Autodesk Inventor part; units mm, degrees
ref_plane "YZ Plane" through (0, 0, 0) normal (1, 0, 0) x (0, 1, 0)
ref_plane "XZ Plane" through (0, 0, 0) normal (0, 1, 0) x (-1, 0, 0)
ref_plane "XY Plane" through (0, 0, 0) normal (0, 0, 1) x (1, 0, 0)
ref_plane "작업 평면1" through (0, 0, 0) normal (0, 0, 1) x (1, 0, 0)
sketch "스케치1" plane through (0, 0, 0) normal (0, 0, 1) x (1, 0, 0)
  line L0 (-20.1, 0.025) -> (-14.5, 0.025)
  line L1 (-20.1, -44.6) -> (-20.1, 8.5)
  line L2 (20.1, 0.025) -> (14.5, 0.025)
  line L3 (20.1, 8.5) -> (20.1, -44.6)
  circle A0 centre (17.3, 4) radius 1.45
  circle A1 centre (-17.3, 4) radius 1.35
  circle A2 centre (-17.3, 4) radius 1.45
  circle A3 centre (17.3, 4) radius 1.55
  line L4 (14.9, 0.025) -> (14.9, 15.025)
  line L5 (-14.9, 15.025) -> (-14.9, 0.025)
  line L6 (-20.1, 0.025) -> (-20.1, 15.025)
  line L7 (20.1, 0.025) -> (20.1, 15.025)
  line L8 (-20.1, 15.025) -> (20.1, 15.025)
  line L9 (-20.1, 0.025) -> (-14.9, 0.025)
  line L10 (14.9, 0.025) -> (20.1, 0.025)
  line L11 (-14.9, 0.025) -> (-14.9, 10.025)
  line L12 (-14.9, 10.025) -> (14.9, 10.025)
  line L13 (14.9, 0.025) -> (20.1, 0.025)
  point P0 (0, 0)
  point P1 (-20.1, 8.5)
  point P2 (-14.9, 0.025)
  dimension "d0" = 0.1
  dimension "d1" = 0.1
  dimension "d4" = 15
  dimension "d5" = 15
  dimension "d9" = 10
extrude "돌출1" add sketch "스케치1" along normal blind 6 contours L1 L6 L8 L5 L0 | L5 L8 L4 L12 | L4 L8 L7 L3 L2
sketch "스케치5" plane through (0, 0, 6) normal (0, 0, 1) x (1, 0, 0)
  line L0 (15, -50.5) -> (11.5, -50.5)
  line L1 (15, -50.5) -> (20.1, -44.5)
  line L2 (20.1, -44.5) -> (20.1, 8.6)
  line L3 (20.1, 8.6) -> (15, 14.6)
  line L4 (15, 14.6) -> (-15, 14.6)
  line L5 (-15, 14.6) -> (-20.1, 8.6)
  line L6 (-20.1, 8.6) -> (-20.1, -44.5)
  line L7 (-20.1, -44.5) -> (-15, -50.5)
  line L8 (-11.5, -50.5) -> (-15, -50.5)
  arc A0 (-14.5, -47.5) -> (-11.5, -50.5) centre (-11.5, -47.5) ccw
  line L9 (-14.5, 6) -> (-14.5, -47.5)
  arc A1 (-11.5, 9) -> (-14.5, 6) centre (-11.5, 6) ccw
  line L10 (11.5, 9) -> (-11.5, 9)
  arc A2 (14.5, 6) -> (11.5, 9) centre (11.5, 6) ccw
  line L11 (14.5, -47.5) -> (14.5, 6)
  arc A3 (11.5, -50.5) -> (14.5, -47.5) centre (11.5, -47.5) ccw
  circle A4 centre (-17.3, -40) radius 1.35
  circle A5 centre (-17.3, -18) radius 1.35
  circle A6 centre (-17.3, 4) radius 1.35
  circle A7 centre (-11, 11.8) radius 1.35
  circle A8 centre (17.3, -40) radius 1.35
  circle A9 centre (17.3, -18) radius 1.35
  circle A10 centre (17.3, 4) radius 1.35
  circle A11 centre (11, 11.8) radius 1.35
  line L12 (20.1, 15.025) -> (-20.1, 15.025)
  line L13 (-20.1, 15.025) -> (-20.1, 0.025)
  line L14 (-20.1, 0.025) -> (-14.9, 0.025)
  line L15 (-14.9, 0.025) -> (-14.9, 10.025)
  line L16 (-14.9, 10.025) -> (14.9, 10.025)
  line L17 (14.9, 10.025) -> (14.9, 0.025)
  line L18 (14.9, 0.025) -> (20.1, 0.025)
  line L19 (20.1, 0.025) -> (20.1, 15.025)
  circle A12 centre (17.3, 4) radius 1.55
  circle A13 centre (-17.3, 4) radius 1.45
  line L20 (-14.9, 15.025) -> (-26.9, 15.025)
  line L21 (-26.9, 15.025) -> (-26.9, -22.7435)
  line L22 (-26.9, -22.7435) -> (-14.9, -22.7435)
  line L23 (-14.9, -22.7435) -> (-14.9, 15.025)
  line L24 (14.9, 15.025) -> (26.9, 15.025)
  line L25 (26.9, 15.025) -> (26.9, -22.7435)
  line L26 (26.9, -22.7435) -> (14.9, -22.7435)
  line L27 (14.9, -22.7435) -> (14.9, 15.025)
  point P0 (0, 0)
  point P1 (0, -36)
  point P2 (20.1, 8.6)
  point P3 (20.1, -22.7435)
  point P4 (-20.1, -22.7435)
  point P5 (-20.1, 15.025)
  point P6 (20.1, 0.025)
  point P7 (-14.9, 0.025)
  dimension "d21" = 12
  dimension "d22" = 12
extrude "돌출5" add sketch "스케치5" against normal blind 6 contours L26 L27 L18 L2 | L23 L22 L6 L14
sketch "스케치12" plane through (0, 0, 6) normal (0, 0, 1) x (1, 0, 0)
  circle A0 centre (-17.3, -18) radius 1.35
  circle A1 centre (17.3, -18) radius 1.35
  line L0 (20.1, 15.025) -> (-20.1, 15.025)
  line L1 (-20.1, 15.025) -> (-20.1, -22.7435)
  line L2 (-20.1, -22.7435) -> (-14.9, -22.7435)
  line L3 (-14.9, -22.7435) -> (-14.9, 10.025)
  line L4 (-14.9, 10.025) -> (14.9, 10.025)
  line L5 (14.9, 10.025) -> (14.9, -22.7435)
  line L6 (14.9, -22.7435) -> (20.1, -22.7435)
  line L7 (20.1, -22.7435) -> (20.1, 15.025)
  circle A2 centre (17.3, 4) radius 1.55
  circle A3 centre (-17.3, 4) radius 1.45
  line L8 (0, 15.025) -> (-5, 15.025)
  line L9 (-5, 15.025) -> (-5, 21.025)
  line L10 (-5, 21.025) -> (0, 21.025)
  line L11 (0, 21.025) -> (0, 15.025)
  line L12 (0, 21.025) -> (5, 21.025)
  line L13 (5, 21.025) -> (5, 15.025)
  line L14 (5, 15.025) -> (0, 15.025)
  line L15 (0, 15.025) -> (0, 21.025)
  point P0 (0, 0)
  point P1 (5, 15.025)
  dimension "d53" = 5
  dimension "d54" = 6
  dimension "d55" = 5
  dimension "d56" = 6
extrude "돌출11" add sketch "스케치12" against normal blind 6 contours L0 L11 L12 L13 | L0 L9 L10 L11
sketch "스케치14" plane through (-20.1, 15.025, 6) normal (0, 1, 0) x (1, 0, 0)
  line L0 (5.2, 6) -> (5.2, 0)
  line L1 (15.1, 0) -> (15.1, 6)
  line L2 (15.1, 6) -> (0, 6)
  line L3 (0, 6) -> (0, 0)
  line L4 (15.1, 0) -> (0, 0)
  line L5 (25.1, 6) -> (25.1, 0)
  line L6 (40.2, 0) -> (25.1, 0)
  line L7 (40.2, 6) -> (40.2, 0)
  line L8 (40.2, 6) -> (25.1, 6)
  line L9 (35, 6) -> (35, 0)
  line L10 (0, 6) -> (2.6, 6)
  circle A0 centre (2.6, 3) radius 1.35
  line L11 (40.2, 6) -> (40.2, 0)
  line L12 (40.2, 6) -> (37.6, 6)
  circle A1 centre (37.6, 3) radius 1.35
  point P0 (20.1, 6)
  dimension "d59" = 6
  dimension "d60" = 5.2
  dimension "d61" = 2.6
  dimension "d62" = 2.7
  dimension "d63" = 2.6
  dimension "d64" = 2.7
extrude "돌출12" cut sketch "스케치14" against normal blind 6 contours A0 | A1
sketch "스케치16" plane through (-20.1, 15.025, 0) normal (-1, 0, 0) x (0, 0, 1)
  line L0 (0, 0) -> (0, -37.7685)
  line L1 (6, -37.7685) -> (0, -37.7685)
  line L2 (6, 0) -> (6, -37.7685)
  line L3 (0, 0) -> (6, 0)
  point P0 (0, -15.025)
extrude "돌출13" add sketch "스케치16" along normal blind 5
sketch "스케치18" plane through (20.1, 15.025, 6) normal (1, 0, 0) x (0, 0, -1)
  line L0 (6, 0) -> (6, -37.7685)
  line L1 (6, 0) -> (0, 0)
  line L2 (0, -37.7685) -> (0, 0)
  line L3 (0, -37.7685) -> (6, -37.7685)
  point P0 (6, -15.025)
extrude "돌출14" add sketch "스케치18" along normal blind 5
move faces "이동1" translate (0, 10, 0) faces at (8.7167, 15.025, 3) (1.6667, 21.025, 4) (-8.7167, 15.025, 3)
sketch "스케치19" plane through (0, 0, 6) normal (0, 0, 1) x (1, 0, 0)
  line L0 (-18.85, 9.025) -> (-16.15, 9.025)
  circle A0 centre (-17.3, 4) radius 1.45
  line L1 (-14.9, 10.025) -> (14.9, 10.025)
  line L2 (-14.9, 10.025) -> (14.9, 10.025)
  circle A1 centre (-17.3, -18) radius 1.35
  circle A2 centre (17.3, -18) radius 1.35
  line L3 (5, 25.025) -> (25.1, 25.025)
  line L4 (5, 25.025) -> (5, 31.025)
  line L5 (5, 31.025) -> (-5, 31.025)
  line L6 (-5, 31.025) -> (-5, 25.025)
  line L7 (-5, 25.025) -> (-25.1, 25.025)
  line L8 (-25.1, -22.7435) -> (-25.1, 25.025)
  line L9 (-25.1, -22.7435) -> (-14.9, -22.7435)
  line L10 (-14.9, -22.7435) -> (-14.9, 10.025)
  line L11 (-14.9, 10.025) -> (14.9, 10.025)
  line L12 (14.9, 10.025) -> (14.9, -22.7435)
  line L13 (14.9, -22.7435) -> (25.1, -22.7435)
  line L14 (25.1, 25.025) -> (25.1, -22.7435)
  circle A3 centre (17.3, 4) radius 1.55
  circle A4 centre (-17.3, 4) radius 1.45
  circle A5 centre (-17.3, -18) radius 1.35
  circle A6 centre (17.3, -18) radius 1.35
  line L15 (25.1, 25.025) -> (5, 25.025)
  line L16 (25.1, -22.7435) -> (25.1, 25.025)
  line L17 (14.9, -22.7435) -> (25.1, -22.7435)
  line L18 (14.9, 10.025) -> (14.9, -22.7435)
  line L19 (-14.9, 10.025) -> (14.9, 10.025)
  line L20 (-14.9, 10.025) -> (-14.9, -22.7435)
  line L21 (-14.9, -22.7435) -> (-25.1, -22.7435)
  line L22 (-25.1, 25.025) -> (-25.1, -22.7435)
  line L23 (-5, 25.025) -> (-25.1, 25.025)
  line L24 (-5, 25.025) -> (-5, 31.025)
  line L25 (-5, 31.025) -> (5, 31.025)
  line L26 (5, 31.025) -> (5, 25.025)
  circle A7 centre (17.3, 4) radius 1.55
  circle A8 centre (-17.3, 4) radius 1.45
  line L27 (-5, 25.025) -> (-5, 31.025)
  line L28 (-14.9, -22.7435) -> (-14.9, 10.025)
  line L29 (-14.9, 10.025) -> (-14.9, -22.7435)
  line L30 (-14.9, 10.025) -> (-14.9, -22.7435)
  line L31 (-14.9, -22.7435) -> (-14.9, 10.025)
  circle A9 centre (-17.3, -18) radius 1.35
  circle A10 centre (-17.3, -18) radius 1.35
  circle A11 centre (-17.3, -18) radius 1.35
  circle A12 centre (-17.3, -18) radius 1.35
  circle A13 centre (-17.3, 4) radius 1.45
  circle A14 centre (-17.3, 4) radius 1.45
  circle A15 centre (-17.3, 4) radius 1.45
  line L32 (-25.1, -22.7435) -> (-14.9, -22.7435)
  line L33 (-14.9, -22.7435) -> (-25.1, -22.7435)
  line L34 (-25.1, -22.7435) -> (-14.9, -22.7435)
  line L35 (-14.9, -22.7435) -> (-25.1, -22.7435)
  line L36 (-25.1, -22.7435) -> (-25.1, 25.025)
  line L37 (-25.1, 25.025) -> (-25.1, -22.7435)
  line L38 (-25.1, 25.025) -> (-25.1, -22.7435)
  line L39 (-25.1, -22.7435) -> (-25.1, 25.025)
  line L40 (14.9, -22.7435) -> (25.1, -22.7435)
  line L41 (14.9, 10.025) -> (14.9, -22.7435)
  line L42 (14.9, 10.025) -> (14.9, -22.7435)
  circle A16 centre (17.3, -18) radius 1.35
  circle A17 centre (17.3, -18) radius 1.35
  circle A18 centre (17.3, 4) radius 1.55
  circle A19 centre (17.3, 4) radius 1.55
  line L43 (16.15, 9.025) -> (18.85, 9.025)
  line L44 (14.9, -22.7435) -> (25.1, -22.7435)
  line L45 (25.1, 25.025) -> (25.1, -22.7435)
  line L46 (25.1, -22.7435) -> (25.1, 25.025)
  line L47 (25.1, -22.7435) -> (25.1, 25.025)
  line L48 (25.1, 25.025) -> (25.1, -22.7435)
  line L49 (-18.85, 9.025) -> (-16.15, 9.025)
  line L50 (-18.85, 25.025) -> (-16.15, 25.025)
  line L51 (-18.85, 9.025) -> (-16.15, 9.025)
  line L52 (-5, 25.025) -> (-25.1, 25.025)
  line L53 (-5, 25.025) -> (-25.1, 25.025)
  line L54 (-18.85, 25.025) -> (-16.15, 25.025)
  line L55 (-5, 25.025) -> (-25.1, 25.025)
  line L56 (-5, 25.025) -> (-25.1, 25.025)
  line L57 (-5, 31.025) -> (-5, 25.025)
  line L58 (5, 31.025) -> (-5, 31.025)
  line L59 (5, 31.025) -> (-5, 31.025)
  line L60 (-5, 31.025) -> (5, 31.025)
  line L61 (-5, 31.025) -> (-5, 25.025)
  line L62 (-5, 25.025) -> (-5, 31.025)
  line L63 (-18.85, 25.025) -> (-16.15, 25.025)
  line L64 (16.15, 25.025) -> (18.85, 25.025)
  line L65 (5, 25.025) -> (25.1, 25.025)
  line L66 (25.1, 25.025) -> (5, 25.025)
  line L67 (5, 31.025) -> (5, 25.025)
  line L68 (5, 25.025) -> (5, 31.025)
  line L69 (5, 25.025) -> (5, 31.025)
  line L70 (5, 31.025) -> (5, 25.025)
  line L71 (-5, 31.025) -> (5, 31.025)
  line L72 (14.9, -22.7435) -> (25.1, -22.7435)
  line L73 (14.9, -22.7435) -> (25.1, -22.7435)
  line L74 (-14.9, 10.025) -> (14.9, 10.025)
  line L75 (-14.9, 10.025) -> (14.9, 10.025)
  circle A20 centre (17.3, -18) radius 1.35
  circle A21 centre (17.3, -18) radius 1.35
  line L76 (14.9, 10.025) -> (14.9, -22.7435)
  line L77 (14.9, 10.025) -> (14.9, -22.7435)
  line L78 (16.15, 9.025) -> (18.85, 9.025)
  line L79 (16.15, 25.025) -> (18.85, 25.025)
  line L80 (16.15, 25.025) -> (18.85, 25.025)
  line L81 (5, 25.025) -> (25.1, 25.025)
  line L82 (25.1, 25.025) -> (5, 25.025)
  circle A22 centre (17.3, 4) radius 1.55
  circle A23 centre (17.3, 4) radius 1.55
  line L83 (16.15, 9.025) -> (18.85, 9.025)
  line L84 (-18.85, 25.025) -> (-18.85, 9.025)
  line L85 (-16.15, 25.025) -> (-16.15, 9.025)
  line L86 (16.15, 25.025) -> (16.15, 9.025)
  line L87 (18.85, 25.025) -> (18.85, 9.025)
  line L88 (-20.1, 15.925) -> (-14.9, 15.925)
  line L89 (-14.9, 15.925) -> (-14.9, 18.125)
  line L90 (-14.9, 18.125) -> (-20.1, 18.125)
  line L91 (-20.1, 18.125) -> (-20.1, 15.925)
  line L92 (-20.1, 15.925) -> (-14.9, 18.125) construction
  line L93 (-14.9, 15.925) -> (-20.1, 18.125) construction
  line L94 (14.9, 15.925) -> (20.1, 15.925)
  line L95 (20.1, 15.925) -> (20.1, 18.125)
  line L96 (20.1, 18.125) -> (14.9, 18.125)
  line L97 (14.9, 18.125) -> (14.9, 15.925)
  line L98 (14.9, 15.925) -> (20.1, 18.125) construction
  line L99 (20.1, 15.925) -> (14.9, 18.125) construction
  point P0 (0, 0)
  point P1 (-17.5, 17.025)
  point P2 (17.5, 17.025)
  dimension "d74" = 5.2
  dimension "d75" = 2.2
  dimension "d76" = 5.2
  dimension "d77" = 2.2
extrude "돌출15" cut sketch "스케치19" against normal blind 10 contours L88 L91 L90 L84 | L84 L90 L85 L88 | L85 L90 L89 L88 | L96 L87 L94 L86 | L86 L94 L97 L96 | L96 L95 L94 L87
properties part number "frame_knee_to_bridge" material "PMMA 플라스틱"
Design review of the part built by this model. Coordinates are the model's own, in mm. A direction names the side the tool comes from. Give positions to 0.01 mm unless a question says otherwise; leave off trailing zeros. Order: outer loops, then holes, each group sorted by start corner. A loop starts at its lowest first (then second) coordinate and runs counter-clockwise, first axis right, second up.
1. Add section A-A, the plane y = -12. State the section outline as (x, z) points.
Solution:
outline: (-25.1, 0) - (-14.9, 0) - (-14.9, 6) - (-25.1, 6) - close; (14.9, 0) - (25.1, 0) - (25.1, 6) - (14.9, 6) - close
2. Tool access review of faces 4 (the flat face through (14.9, -7, 3)), 5 (the flat face through (25.1, 1, 3)), 6 (the flat face through (-14.9, 17, 3)), 7 (the flat face through (-18, 9.025, 3)): name each direction out of +Z, -Z, +X, -X, +Y, -Y from which nothing blocks a thin tool from reaching the whole face with its end or side.
Solution:
face 4: +Z, -Z, -Y
face 5: +Z, -Z, +X, +Y, -Y
face 6: +Z, -Z
face 7: +Y
3. Mouldability with a two-part tool opening along Y and no side actions: class faces 1 (the flat face through (-19, 15.925, 4)), 2 (the flat face through (5, 28, 3)), 3 (the flat face through (0, 31.025, 3)) as +Y half, -Y half, draft (parallel to the pull), parting line (faces both ways), or undercut.
Solution:
face 1: undercut
face 2: draft
face 3: +Y half
4. Add section C-C, the plane y = 4. State the section outline as (x, z) points, then the cut area to 3 significant figures.
Solution:
outline: (-25.1, 0) - (-18.75, 0) - (-18.75, 6) - (-25.1, 6) - close; (-15.85, 0) - (-14.9, 0) - (-14.9, 6) - (-15.85, 6) - close; (14.9, 0) - (15.75, 0) - (15.75, 6) - (14.9, 6) - close; (18.85, 0) - (25.1, 0) - (25.1, 6) - (18.85, 6) - close
area: 86.4 mm2
5. For pin 1 Ø3 at (x, z) = (17.5, 3) entering from +Y (3 decimals); pin 2 Ø3 at (x, z) = (-3, 4) entering from -Y (3 decimals); pin 3 Ø0.8 at (x, z) = (-18, 3) entering from +Y (3 decimals), all flat-tipped, find the tip position at first contact; note any pin that passes through.
Solution:
pin 1: stops at y = 25.025
pin 2: stops at y = 10.025
pin 3: stops at y = 9.025
6. To check wall thickness, follow L1, parallel to X at y = 13.5, z = 3; L2, parallel to X at y = 4, z = 2.95; L3, parallel to X at y = -8.5, z = 2.1. State the ranges of each line that lie inside material, in increasing order.
Solution:
L1: x = -25.1 to -18.85, -16.15 to 16.15, 18.85 to 25.1
L2: x = -25.1 to -18.75, -15.85 to -14.9, 14.9 to 15.75, 18.85 to 25.1
L3: x = -25.1 to -14.9, 14.9 to 25.1
7. Add section B-B, the plane x = -17.5. State how many separate pieces and enclosed holes the cut face has, then the cut area to 3 significant figures.
Solution:
separate pieces: 5
enclosed holes: 0
area: 203 mm2
